Check sheet for the modelled part. Datum: model origin and axes. Units: mm. Face numbers are marked on the shaded views. A direction names the side the tool comes from. Round coordinates to 2 decimals unless told otherwise and drop trailing zeros. Write each loop counter-clockwise with the first axis right and the second up, starting at its lowest first coordinate (ties: lowest second). Pieces come first, ordered by that corner, then holes.
Item 1: Material ranges on line 1 along Z through (x, y) = (28, 7.5); line 2 along X through (y, z) = (10.5, 0); line 3 along X through (y, z) = (4, 6.5), recorded low to high.
Item 2: Set-up check for the marked faces 4 and 5: record each of +Z, -Z, +X, -X, +Y, -Y from which the full face is reachable in a straight line by a thin tool's end or side.
Item 3: Section check A-A, the plane y = 2. Record the cut outline in (x, z), plus the area to 3 significant figures.
Item 4: Release check for a two-part mould opening along Z. For the marked faces 1, 2 and 3 record: pulls with the +Z half, pulls with the -Z half, needs draft (parallel to the pull), parting line crosses it, or undercut.
Item 5: Section check B-B, the plane x = -36. Record the cut outline in (y, z).
Item 6: Section check C-C, the plane z = -5.5. Record the cut outline in (x, y).
from build123d import *

# Parameters (mm, degrees)
BOSS_EXTRUDE1_DEPTH      = 25
BOSS_EXTRUDE1_DEPTH_BACK = 25
SKETCH1_W                = 100
SKETCH1_H                = 38.5
SKETCH1_W_2              = 80
SKETCH1_H_2              = 18.5
BOSS_EXTRUDE2_DEPTH      = 25
BOSS_EXTRUDE2_DEPTH_BACK = 25
SKETCH2_R                = 5


with BuildPart() as part:
    # Sketch1 → Boss-Extrude1 (new, two sides: drawn at the far end of the back side and taken through both)
    with BuildSketch(Plane(origin=(0, 0, 0), x_dir=(1, 0, 0), z_dir=(0, 1, 0)).offset(-BOSS_EXTRUDE1_DEPTH_BACK)):
        Rectangle(SKETCH1_W, SKETCH1_H)
        Rectangle(SKETCH1_W_2, SKETCH1_H_2, mode=Mode.SUBTRACT)
    extrude(amount=BOSS_EXTRUDE1_DEPTH + BOSS_EXTRUDE1_DEPTH_BACK)

    # Sketch2 → Boss-Extrude2 (add, two sides: drawn at the far end of the back side and taken through both)
    with BuildSketch(Plane(origin=(0, 0, 0), x_dir=(1, 0, 0), z_dir=(0, 1, 0)).offset(-BOSS_EXTRUDE2_DEPTH_BACK)):
        with Locations((40, 9.25)):
            Circle(SKETCH2_R)
        with Locations((40, -9.25)):
            Circle(SKETCH2_R)
        with Locations((-40, 9.25)):
            Circle(SKETCH2_R)
        with Locations((-40, -9.25)):
            Circle(SKETCH2_R)
    extrude(amount=BOSS_EXTRUDE2_DEPTH + BOSS_EXTRUDE2_DEPTH_BACK)


solid = part.part
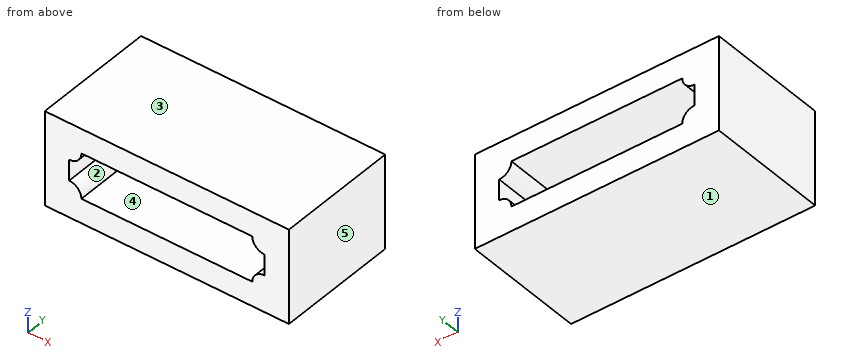
Values found:
1. line 1: z = -19.25 to -9.25, 9.25 to 19.25
1. line 2: x = -50 to -40, 40 to 50
1. line 3: x = -50 to -35.82, 35.82 to 50
2. face 4: +Y, -Y
2. face 5: +Z, -Z, +X, +Y, -Y
3. outline: (-50, -19.25) - (50, -19.25) - (50, 19.25) - (-50, 19.25) - close; hole (-40, -4.25) arc R5 cw to (-35, -9.25) - (35, -9.25) arc R5 cw to (40, -4.25) - (40, 4.25) arc R5 cw to (35, 9.25) - (-35, 9.25) arc R5 cw to (-40, 4.25) - close
3. area: 2,450 mm2
4. face 1: pulls with the -Z half
4. face 2: undercut
4. face 3: pulls with the +Z half
5. outline: (-25, -19.25) - (25, -19.25) - (25, -6.25) - (-25, -6.25) - close; (-25, 6.25) - (25, 6.25) - (25, 19.25) - (-25, 19.25) - close
6. outline: (-50, -25) - (-36.69, -25) - (-36.69, 25) - (-50, 25) - close; (36.69, -25) - (50, -25) - (50, 25) - (36.69, 25) - close
